Read the model definition and answer for the solid it produces. Units are mm, in the model's axes. A direction names the side the tool comes from. Coordinates: 2 decimals unless noted, no trailing zeros. Write each loop counter-clockwise with the first axis right and the second up, starting at its lowest first coordinate (ties: lowest second). Pieces come first, ordered by that corner, then holes.
(1) Determine the mould class of faces 3 (the flat face through (3.13, -77.68, 237.06)), 4 (the cylindrical face through (3.219, -14.702, 225.856)), 5 (the flat face through (3.175, 141, 287)), 6 (the flat face through (3.131, 162.031, 287.426)) for opening direction Y: pulls with the +Y half, pulls with the -Y half, needs draft (parallel to the pull), parting line crosses it, or undercut.
(2) The part is cut by section C-C, the plane z = 202. Determine the outline of the cut face in (x, y), and give its area (3 significant figures).
(3) The part is cut by section D-D, the plane y = -125.5. Determine the outline of the cut face in (x, z), and give its area (3 significant figures).
(4) Which of the six approach directions +Z, -Z, +X, -X, +Y, -Y give full straight-line access (tool end or side, diameter ignored) to faces 1 (the cylindrical face through (4.785, 115.861, 270.765)), 2 (the cylindrical face through (3.131, -164.602, 159.058))?
(5) The part is cut by section A-A, the plane y = 165.1. Determine the outline of the cut face in (x, z).
(6) Given pin 1 (6.5 mm diameter, centred on y = 143.62, z = 279.53, fed in from +X) (3 decimals); pin 2 (3 mm diameter, centred on x = 4, y = 132.5, fed in from -Z), each flat-ended and moving along its own axis, determine where each tip first touches the part or whether it passes through.
(7) Straight lines are drawn through the part: line 1 along Z through (x, y) = (1.5, 142); line 2 along Y through (x, z) = (2.5, 286); line 3 along Y through (x, z) = (5, 298). For each, find the intervals that lie inside material, in ascending order.
(8) The part is cut by section B-B, the plane x = 4.75. Determine the outline of the cut face in (y, z) (1 decimal), and give its area (3 significant figures).
Autodesk Inventor part; units mm, degrees
ref_plane "YZ Plane" through (0, 0, 0) normal (1, 0, 0) x (0, 1, 0)
ref_plane "XZ Plane" through (0, 0, 0) normal (0, 1, 0) x (-1, 0, 0)
ref_plane "XY Plane" through (0, 0, 0) normal (0, 0, 1) x (1, 0, 0)
sketch "Sketch1" plane through (0, 0, 0) normal (1, 0, 0) x (0, 1, 0)
  circle A0 centre (0, 0) radius 203.2 construction
  circle A1 centre (165.1, 167.1631) radius 38.1 construction
  circle A2 centre (165.1, 167.1631) radius 31.75 construction
  circle A3 centre (-177.8, 153.586) radius 38.1 construction
  circle A4 centre (-177.8, 153.586) radius 31.75 construction
  circle A5 centre (279.4, 30.6697) radius 38.1 construction
  circle A6 centre (279.4, 30.6697) radius 31.75 construction
  line L0 (371.6722, 159.6086) -> (293.9242, 243.3925) construction
  line L1 (293.9242, 243.3925) -> (72.8278, 38.2242) construction
  line L2 (72.8278, 38.2242) -> (150.5758, -45.5597) construction
  line L3 (150.5758, -45.5597) -> (371.6722, 159.6086) construction
  line L4 (371.6722, 159.6086) -> (72.8278, 38.2242) construction
  line L5 (293.9242, 243.3925) -> (150.5758, -45.5597) construction
  line L6 (165.1, 167.1631) -> (279.4, 30.6697) construction
  point P0 (222.25, 98.9164)
  dimension "d0" = 406.4
  dimension "d1" = 76.2
  dimension "d2" = 6.35
  dimension "d4" = 114.3
  dimension "d5" = 301.625
  dimension "d6" = 177.8
  dimension "d51" = 165.1
  dimension "d52" = 279.4
  dimension "d53" = 30.6697
sketch "Sketch4" plane through (0, 0, 0) normal (1, 0, 0) x (0, 1, 0)
  circle A0 centre (0, 0) radius 203.2 construction
  circle A1 centre (165.1, 167.1631) radius 38.1 construction
  circle A2 centre (165.1, 167.1631) radius 31.75 construction
  circle A3 centre (-177.8, 153.586) radius 38.1 construction
  circle A4 centre (-177.8, 153.586) radius 31.75 construction
  circle A5 centre (279.4, 30.6697) radius 38.1 construction
  circle A6 centre (279.4, 30.6697) radius 31.75 construction
  line L0 (371.6722, 159.6086) -> (293.9242, 243.3925) construction
  line L1 (293.9242, 243.3925) -> (72.8278, 38.2242) construction
  line L2 (72.8278, 38.2242) -> (150.5758, -45.5597) construction
  line L3 (150.5758, -45.5597) -> (371.6722, 159.6086) construction
  line L4 (371.6722, 159.6086) -> (72.8278, 38.2242) construction
  line L5 (293.9242, 243.3925) -> (150.5758, -45.5597) construction
  line L6 (165.1, 167.1631) -> (279.4, 30.6697) construction
  circle A7 centre (-177.8, 153.586) radius 14.2875
  circle A8 centre (165.1, 167.1631) radius 14.2875
  circle A9 centre (279.4, 30.6697) radius 14.2875
  circle A10 centre (165.1, 167.1631) radius 23.8125 construction
  circle A11 centre (279.4, 30.6697) radius 23.8125 construction
  circle A12 centre (-177.8, 153.586) radius 23.8125 construction
  line L7 (261.1433, 15.3815) -> (146.8433, 151.8749)
  line L8 (309.92, 115.3835) -> (248.7672, 188.4102)
  line L9 (309.92, 115.3835) -> (303.1398, 28.8105)
  line L10 (248.7672, 188.4102) -> (130.1238, 323.85)
  line L11 (130.1238, 323.85) -> (31.75, 298.45)
  line L12 (31.75, 298.45) -> (-189.4509, 174.3536)
  arc A13 (148.3669, 150.2209) -> (-159.7797, 138.0199) centre (0, 0) ccw
  arc A14 (148.3669, 150.2209) -> (146.8433, 151.8749) centre (165.1, 167.1631) ccw
  arc A15 (256.4562, 24.2964) -> (303.1398, 28.8105) centre (279.4, 30.6697) ccw
  line L13 (332.7982, 201.5005) -> (111.7018, -3.6678) construction
  arc A16 (-189.4509, 174.3536) -> (-159.7797, 138.0199) centre (-177.8, 153.586) ccw
  point P0 (222.25, 98.9164)
  point P1 (279.3436, 151.8969)
  point P2 (261.1433, 15.3815)
  point P3 (147.5854, 150.9888)
  dimension "d27" = 28.575
  dimension "d29" = 9.525
  dimension "d31" = 101.6
  dimension "d33" = 101.6
  dimension "d35" = 95.25
  dimension "d58" = 298.45
  dimension "d59" = 323.85
  dimension "d60" = 31.75
extrude "Extrusion2" add sketch "Sketch4" along normal blind 6.35 contours L7 A14 A13 | L7 A13 A16 L12 L11 L10 L8 L9 A15
sketch "Sketch5" plane through (6.35, 0, 0) normal (1, 0, 0) x (0, 0, -1)
  line L0 (-323.85, 130.1238) -> (-298.45, 31.75)
  line L1 (-301.2085, 93.2336) -> (-294.8585, 68.6402) construction
  point P0 (0, 0)
  point P1 (-298.0335, 80.9369)
  point P2 (-311.15, 80.9369)
  point P3 (-298.0335, 80.9369)
  point P4 (-311.15, 80.9369)
  dimension "d39" = 12.7
  dimension "d57" = 25.4
hole "Hole2" at (6.35, 93.2336, 301.2085) at (6.35, 80.9369, 298.0335) at (6.35, 68.6402, 294.8585) direction (-1, 0, 0) diameter 5.1054 end through all
sketch "Sketch6" plane through (6.35, 0, 0) normal (1, 0, 0) x (0, 0, -1)
  circle A0 centre (-298.0335, 80.9369) radius 2.5527
  circle A1 centre (-301.2085, 93.2336) radius 2.5527
  circle A2 centre (-294.8585, 68.6402) radius 2.5527
  arc A3 (-15.3815, 261.1433) -> (-28.8105, 303.1398) centre (-30.6697, 279.4) ccw
  line L0 (-28.8105, 303.1398) -> (-115.3835, 309.92)
  line L1 (-115.3835, 309.92) -> (-188.4102, 248.7672)
  line L2 (-188.4102, 248.7672) -> (-323.85, 130.1238)
  line L3 (-323.85, 130.1238) -> (-298.45, 31.75)
  line L4 (-298.45, 31.75) -> (-174.3536, -189.4509)
  arc A4 (-174.3536, -189.4509) -> (-138.0199, -159.7797) centre (-153.586, -177.8) ccw
  arc A5 (-150.9888, 147.5854) -> (-138.0199, -159.7797) centre (0, 0) ccw
  line L5 (-150.9888, 147.5854) -> (-15.3815, 261.1433)
  circle A6 centre (-30.6697, 279.4) radius 14.2875
  circle A7 centre (-167.1631, 165.1) radius 14.2875
  circle A8 centre (-153.586, -177.8) radius 14.2875
  circle A9 centre (-167.1631, 165.1) radius 26.9875 construction
  line L6 (-167.1631, 192.0875) -> (-253.1141, 192.0875)
  line L7 (-188.4102, 248.7672) -> (-323.85, 130.1238) construction
  circle A10 centre (-167.1631, 165.1) radius 14.2875 construction
  line L8 (-150.9888, 147.5854) -> (-15.3815, 261.1433) construction
  arc A11 (-142.138, 154.997) -> (-167.1631, 192.0875) centre (-167.1631, 165.1) ccw
  dimension "d65" = 12.7
extrude "Extrusion3" cut sketch "Sketch6" against normal blind 25.4 contours A0 | A1 | A2 | L5 A11 L6 L2 L1 L0 A3 | A8
fillet "Fillet1" radius 6.604 4 edges at (3.175, 192.0875, 253.1141) (3.175, 130.1238, 323.85) (3.175, 31.75, 298.45) (3.175, 154.997, 142.138)
sketch "Sketch8" plane through (6.35, 0, 0) normal (1, 0, 0) x (0, 0, -1)
  circle A0 centre (-283.6185, 131.5988) radius 7.6454 construction
  circle A1 centre (-283.6185, 131.5988) radius 19.05 construction
  circle A2 centre (-167.1631, 165.1) radius 28.6512 construction
  arc A3 (-320.7904, 132.804) -> (-322.8331, 126.1854) centre (-316.4388, 127.8364) ccw construction
  line L0 (-320.7904, 132.804) -> (-254.9821, 190.4511) construction
  arc A4 (-250.6306, 192.0875) -> (-254.9821, 190.4511) centre (-250.6306, 185.4835) ccw construction
  line L1 (-250.6306, 192.0875) -> (-167.1631, 192.0875) construction
  arc A5 (-141.4456, 156.9185) -> (-167.1631, 192.0875) centre (-167.1631, 165.1) ccw construction
  arc A6 (-143.4989, 153.8574) -> (-141.4456, 156.9185) centre (-147.7388, 158.9206) ccw construction
  line L2 (-143.4989, 153.8574) -> (-150.9888, 147.5854) construction
  arc A7 (-150.9888, 147.5854) -> (-138.0199, -159.7797) centre (0, 0) ccw construction
  arc A8 (-174.3536, -189.4509) -> (-138.0199, -159.7797) centre (-153.586, -177.8) ccw construction
  line L3 (-174.3536, -189.4509) -> (-298.0299, 31.0012) construction
  arc A9 (-298.6647, 32.5814) -> (-298.0299, 31.0012) centre (-292.2704, 34.2324) ccw construction
  line L4 (-298.6647, 32.5814) -> (-322.8331, 126.1854) construction
  circle A10 centre (-298.0335, 80.9369) radius 2.5527 construction
  circle A11 centre (-301.2085, 93.2336) radius 2.5527 construction
  circle A12 centre (-294.8585, 68.6402) radius 2.5527 construction
  circle A13 centre (-153.586, -177.8) radius 14.2875 construction
  circle A14 centre (-167.1631, 165.1) radius 14.2875 construction
  circle A15 centre (-283.6185, 131.5988) radius 9.525
  circle A16 centre (-167.1631, 165.1) radius 14.2875
  circle A17 centre (-247.5393, 27.9128) radius 14.2875
  circle A18 centre (-247.5393, 27.9128) radius 19.05 construction
  circle A19 centre (-239.0544, -9.2303) radius 19.05 construction
  circle A20 centre (-239.0544, -9.2303) radius 14.2875
  dimension "d76" = 15.2908
  dimension "d77" = 38.1
  dimension "d78" = 57.3024
  dimension "d79" = 121.1783
  dimension "d81" = 25.4
  dimension "d83" = 19.05
  dimension "d84" = 28.575
  dimension "d85" = 158.9989
  dimension "d87" = 38.1
  dimension "d88" = 188.9989
  dimension "d111" = 31.75
extrude "Extrusion4" cut sketch "Sketch8" against normal through all
sketch "Sketch9" plane through (6.35, 0, 0) normal (1, 0, 0) x (0, 0, -1)
  circle A0 centre (-247.5393, 27.9128) radius 14.2875 construction
  circle A1 centre (-283.6185, 131.5988) radius 9.525 construction
  circle A2 centre (-239.0544, -9.2303) radius 14.2875 construction
  circle A3 centre (-167.1631, 165.1) radius 14.2875 construction
  arc A4 (-320.7904, 132.804) -> (-322.8331, 126.1854) centre (-316.4388, 127.8364) ccw construction
  line L0 (-320.7904, 132.804) -> (-254.9821, 190.4511) construction
  arc A5 (-250.6306, 192.0875) -> (-254.9821, 190.4511) centre (-250.6306, 185.4835) ccw construction
  line L1 (-250.6306, 192.0875) -> (-167.1631, 192.0875) construction
  arc A6 (-141.4456, 156.9185) -> (-167.1631, 192.0875) centre (-167.1631, 165.1) ccw construction
  arc A7 (-143.4989, 153.8574) -> (-141.4456, 156.9185) centre (-147.7388, 158.9206) ccw construction
  line L2 (-143.4989, 153.8574) -> (-150.9888, 147.5854) construction
  arc A8 (-150.9888, 147.5854) -> (-138.0199, -159.7797) centre (0, 0) ccw construction
  arc A9 (-174.3536, -189.4509) -> (-138.0199, -159.7797) centre (-153.586, -177.8) ccw construction
  line L3 (-174.3536, -189.4509) -> (-298.0299, 31.0012) construction
  arc A10 (-298.6647, 32.5814) -> (-298.0299, 31.0012) centre (-292.2704, 34.2324) ccw construction
  line L4 (-298.6647, 32.5814) -> (-322.8331, 126.1854) construction
  circle A11 centre (-298.0335, 80.9369) radius 2.5527 construction
  circle A12 centre (-301.2085, 93.2336) radius 2.5527 construction
  circle A13 centre (-294.8585, 68.6402) radius 2.5527 construction
  circle A14 centre (-153.586, -177.8) radius 14.2875 construction
  circle A15 centre (-283.6185, 131.5988) radius 20.32
  line L5 (-284.5175, 151.8989) -> (-290.8021, 159.0733)
  line L6 (-303.6236, 135.1623) -> (-309.9082, 142.3366)
  line L7 (-254.9821, 190.4511) -> (-320.7904, 132.804) construction
  line L8 (-290.8021, 159.0733) -> (-309.9082, 142.3366) construction
  line L9 (-283.6185, 131.5988) -> (-300.3551, 150.7049) construction
  line L10 (-290.8021, 159.0733) -> (-309.9082, 142.3366)
  dimension "d93" = 40.64
  dimension "d96" = 25.4
extrude "Extrusion5" cut sketch "Sketch9" against normal blind 3.175
sketch "Sketch10" plane through (3.175, 0, 0) normal (1, 0, 0) x (0, 0, -1)
  circle A0 centre (-247.5393, 27.9128) radius 14.2875 construction
  circle A1 centre (-283.6185, 131.5988) radius 9.525 construction
  circle A2 centre (-239.0544, -9.2303) radius 14.2875 construction
  circle A3 centre (-167.1631, 165.1) radius 14.2875 construction
  arc A4 (-298.6647, 32.5814) -> (-298.0299, 31.0012) centre (-292.2704, 34.2324) ccw construction
  line L0 (-298.6647, 32.5814) -> (-322.8331, 126.1854) construction
  arc A5 (-320.7904, 132.804) -> (-322.8331, 126.1854) centre (-316.4388, 127.8364) ccw construction
  line L1 (-320.7904, 132.804) -> (-309.9082, 142.3366) construction
  line L2 (-309.9082, 142.3366) -> (-303.6236, 135.1623) construction
  arc A6 (-303.6236, 135.1623) -> (-284.5175, 151.8989) centre (-283.6185, 131.5988) ccw construction
  line L3 (-284.5175, 151.8989) -> (-290.8021, 159.0733) construction
  line L4 (-290.8021, 159.0733) -> (-254.9821, 190.4511) construction
  arc A7 (-250.6306, 192.0875) -> (-254.9821, 190.4511) centre (-250.6306, 185.4835) ccw construction
  line L5 (-250.6306, 192.0875) -> (-167.1631, 192.0875) construction
  arc A8 (-141.4456, 156.9185) -> (-167.1631, 192.0875) centre (-167.1631, 165.1) ccw construction
  arc A9 (-143.4989, 153.8574) -> (-141.4456, 156.9185) centre (-147.7388, 158.9206) ccw construction
  line L6 (-143.4989, 153.8574) -> (-150.9888, 147.5854) construction
  arc A10 (-150.9888, 147.5854) -> (-138.0199, -159.7797) centre (0, 0) ccw construction
  arc A11 (-174.3536, -189.4509) -> (-138.0199, -159.7797) centre (-153.586, -177.8) ccw construction
  line L7 (-174.3536, -189.4509) -> (-298.0299, 31.0012) construction
  line L8 (-309.9082, 142.3366) -> (-290.8021, 159.0733) construction
  circle A12 centre (-298.0335, 80.9369) radius 2.5527 construction
  circle A13 centre (-301.2085, 93.2336) radius 2.5527 construction
  circle A14 centre (-294.8585, 68.6402) radius 2.5527 construction
  circle A15 centre (-153.586, -177.8) radius 14.2875 construction
  circle A16 centre (-283.6185, 131.5988) radius 12.7 construction
  point P0 (-279.5294, 143.6226)
  point P1 (-291.9868, 141.1519)
  point P2 (-296.0758, 129.1282)
  point P3 (-287.7075, 119.5751)
  point P4 (-275.2501, 122.0458)
  point P5 (-271.1611, 134.0695)
  dimension "d97" = 25.4
  dimension "d100" = 360
  dimension "d110" = 19.05
hole "Hole4" at (3.175, 143.6226, 279.5294) at (3.175, 141.1519, 291.9868) at (3.175, 129.1282, 296.0758) at (3.175, 119.5751, 287.7075) at (3.175, 122.0458, 275.2501) at (3.175, 134.0695, 271.1611) direction (-1, 0, 0) diameter 5.1054 end through all
properties part number "GP4-001" material "Polycarbonate, Smoke"
Computed:
1. face 3: pulls with the -Y half
1. face 4: undercut
1. face 5: undercut
1. face 6: pulls with the +Y half
2. outline: (0, -140.17) - (6.35, -140.17) - (6.35, -61.44) - (0, -61.44) - close; (0, 61.44) - (6.35, 61.44) - (6.35, 192.09) - (0, 192.09) - close
2. area: 1,330 mm2
3. outline: (0, 169.79) - (6.35, 169.79) - (6.35, 210.23) - (0, 210.23) - close
3. area: 257 mm2
4. face 1: +X
4. face 2: +X, -X
5. outline: (0, 140.18) - (6.35, 140.18) - (6.35, 152.88) - (0, 152.88) - close; (0, 181.45) - (6.35, 181.45) - (6.35, 283.92) - (0, 283.92) - close
6. pin 1: stops at x = 3.175
6. pin 2: stops at z = 163.17
7. line 1: z = 156.25 to 277.56, 281.5 to 289.58, 294.39 to 310.29
7. line 2: y = 9.56 to 117.68, 121.47 to 122.38, 140.82 to 163.28
7. line 3: y = 30.95 to 78.38, 83.49 to 117.24
8. outline: (-189.5, 174.4) arc R23.8 ccw (long way) to (-159.8, 138) arc R211.1 cw to (147.6, 151) - (153.9, 143.5) arc R6.6 ccw to (156.9, 141.4) arc R27 ccw to (192.1, 167.2) - (192.1, 250.6) arc R6.6 ccw to (190.5, 255) - (159.1, 290.8) - (151.9, 284.5) arc R20.3 cw (long way) to (135.2, 303.6) - (142.3, 309.9) - (132.8, 320.8) arc R6.6 ccw to (126.2, 322.8) - (32.6, 298.7) arc R6.6 ccw to (31, 298) - close; hole circle Ø28.6 at (-177.8, 153.6); hole circle Ø28.6 at (-9.2, 239.1); hole circle Ø28.6 at (27.9, 247.5); hole circle Ø5.1 at (68.6, 294.9); hole circle Ø5.1 at (80.9, 298); hole circle Ø5.1 at (93.2, 301.2); hole circle Ø28.6 at (165.1, 167.2)
8. area: 28,100 mm2
